Part model, mm, in its own coordinate system. A direction names the side the tool comes from. Give positions to 0.01 mm unless a question says otherwise; leave off trailing zeros. Order: outer loops, then holes, each group sorted by start corner. A loop starts at its lowest first (then second) coordinate and runs counter-clockwise, first axis right, second up. Notation, with made-up numbers: (-16, -5.5) -> (41, -5.5) arc R16 ccw to (41, 13.5) -> close; hole circle Ø1 at (35.5, 2.25). An arc over 180 degrees is marked (long way). Write item = value, one per line. Start each with the question number.
Item 1: Drill centre lines: line 1 along Z through (x, y) = (205.5, 1); line 2 along X through (y, z) = (9.1, 0). Where is each one in solid material? Low to high.
Item 2: Tool access for faces 5 (the face through (262, -9, 0)), 6 (the face through (-4, -8, 0)), 7 (the face through (-253.37, 9.01, -1.19)): list every direction of +Z, -Z, +X, -X, +Y, -Y with a clear straight run to the whole face (end or side of a thin tool).
Item 3: Band-saw the part on B-B on x = 24.5. Write the cut outline in (y, z).
Item 4: Pull direction Y, two halves, no side cores. Call faces 1 (the face through (-4, 0, 8)), 2 (the face through (-4, 8, 0)), 3 (the face through (-4, -10, 0)), 4 (the face through (-4, 0, -10)): +Y half, -Y half, draft (parallel to the pull), parting line (faces both ways), or undercut.
Item 5: Band-saw the part on A-A on y = -3.5. Write the cut outline in (x, z), plus the area to 3 significant figures.
```python
from build123d import *

# Parameters (mm, degrees)
F_20_X_20_X_2_1_DEPTH = 524
CUT_EXTRUDE_1_REACH   = 264.952
SKETCH_3_R            = 5.5
SKETCH_4_R            = 2.5
CUT_EXTRUDE_2_DEPTH   = 263.807914645


with BuildPart() as part:
    # Sketch1 → Квадратная труба 20 X 20 X 2(1) (new body)
    with BuildSketch(Plane.YZ.offset(-262)):
        with BuildLine():
            Line((-7, -10), (7, -10))
            ThreePointArc((7, -10), (9.121320344, -9.121320344), (10, -7))
            Line((10, -7), (10, 7))
            ThreePointArc((10, 7), (9.121320344, 9.121320344), (7, 10))
            Line((7, 10), (-7, 10))
            ThreePointArc((-7, 10), (-9.121320344, 9.121320344), (-10, 7))
            Line((-10, 7), (-10, -7))
            ThreePointArc((-10, -7), (-9.121320344, -9.121320344), (-7, -10))
        make_face()
        with BuildLine():
            Line((-7, -8), (7, -8))
            ThreePointArc((7, -8), (7.707106781, -7.707106781), (8, -7))
            Line((8, -7), (8, 7))
            ThreePointArc((8, 7), (7.707106781, 7.707106781), (7, 8))
            Line((7, 8), (-7, 8))
            ThreePointArc((-7, 8), (-7.707106781, 7.707106781), (-8, 7))
            Line((-8, 7), (-8, -7))
            ThreePointArc((-8, -7), (-7.707106781, -7.707106781), (-7, -8))
        make_face(mode=Mode.SUBTRACT)
    extrude(amount=F_20_X_20_X_2_1_DEPTH)

    # Эскиз3 → Вырез-Вытянуть1 (cut, up to next)
    with BuildSketch(Plane(origin=(0, 10, 0), x_dir=(1, 0, 0), z_dir=(0, 1, 0)), mode=Mode.PRIVATE) as cut_extrude_1_sk1:
        with Locations(Location((-248, 0, 0), (0, 0, 270))):
            Circle(SKETCH_3_R)
    cut_extrude_1_tool1 = extrude(cut_extrude_1_sk1.sketch, amount=-CUT_EXTRUDE_1_REACH, mode=Mode.PRIVATE) & part.part
    # Эскиз3 → Вырез-Вытянуть1 (cut, up to next)
    with BuildSketch(Plane(origin=(0, 10, 0), x_dir=(1, 0, 0), z_dir=(0, 1, 0)), mode=Mode.PRIVATE) as cut_extrude_1_sk2:
        with Locations(Location((248, 0, 0), (0, 0, 270))):
            Circle(SKETCH_3_R)
    cut_extrude_1_tool2 = extrude(cut_extrude_1_sk2.sketch, amount=-CUT_EXTRUDE_1_REACH, mode=Mode.PRIVATE) & part.part
    add(cut_extrude_1_tool1.solids().sort_by_distance((-248, 10, 0))[0], mode=Mode.SUBTRACT)
    add(cut_extrude_1_tool2.solids().sort_by_distance((248, 10, 0))[0], mode=Mode.SUBTRACT)

    # Эскиз4 → Вырез-Вытянуть2 (cut, through all)
    with BuildSketch(Plane(origin=(0, -8, 0), x_dir=(1, 0, 0), z_dir=(0, 1, 0))):
        with Locations(Location((-248, 0, 0), (0, 0, 270))):
            Circle(SKETCH_4_R)
        with Locations(Location((248, 0, 0), (0, 0, 270))):
            Circle(SKETCH_4_R)
    extrude(amount=-CUT_EXTRUDE_2_DEPTH, mode=Mode.SUBTRACT)


solid = part.part
```
Values found:
q1.line_1 = -10 to -8, 8 to 10
q1.line_2 = -262 to -253.5, -242.5 to 242.5, 253.5 to 262
q2.face_5 = +Z, -Z, +X, +Y, -Y
q2.face_6 = +X, -X
q2.face_7 = +Y
q3.outline = (-10, -7) arc R3 ccw to (-7, -10) -> (7, -10) arc R3 ccw to (10, -7) -> (10, 7) arc R3 ccw to (7, 10) -> (-7, 10) arc R3 ccw to (-10, 7) -> close; hole (-8, -7) arc R1 ccw to (-7, -8) -> (7, -8) arc R1 ccw to (8, -7) -> (8, 7) arc R1 ccw to (7, 8) -> (-7, 8) arc R1 ccw to (-8, 7) -> close
q4.face_1 = undercut
q4.face_2 = undercut
q4.face_3 = -Y half
q4.face_4 = draft
q5.outline = (-262, -10) -> (262, -10) -> (262, -8) -> (-262, -8) -> close; (-262, 8) -> (262, 8) -> (262, 10) -> (-262, 10) -> close
q5.area = 2,100 mm^2
